Source: three-view drawing plus pictorial views. Frame: mm from the lowest corner of the part. A direction names the side the tool comes from. Give positions to 0.01 mm unless a question says otherwise; leave off trailing zeros. Order: outer loops, then holes, each group sorted by start corner. A loop starts at its lowest first (then second) coordinate and runs counter-clockwise, first axis right, second up. Notation, with made-up numbers: (56, 66) -> (95, 66) arc R21 ccw to (95, 73) -> close; hole circle Ø7 at (74.5, -12). An arc over 180 degrees is marked (long way). Write item = value, one per line.
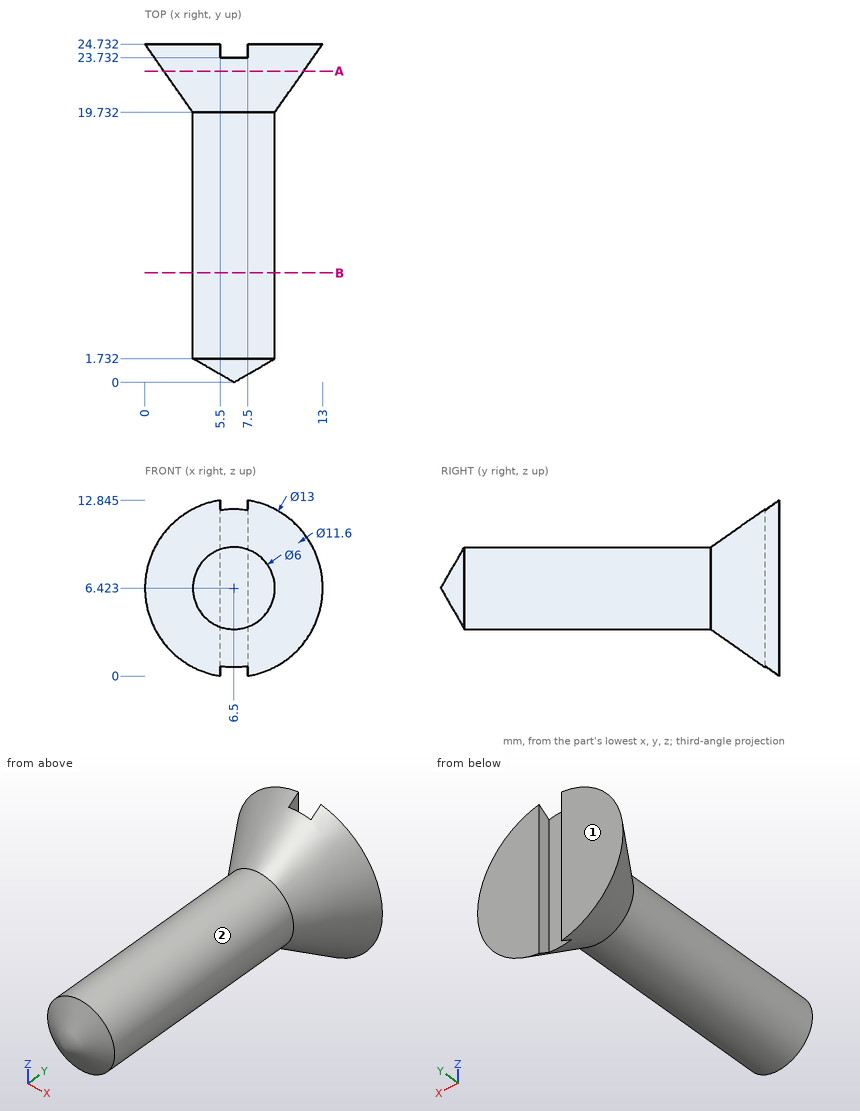
1) First-contact query: P1, Ø0.5, axis at y = 24.5, z = 4, coming from the -X side; P2, Ø5, axis at y = 13.5, z = 6, coming from the -X side; P3, Ø1.1, axis at y = 24, z = 5.5, coming from the +X side; P4, Ø5, axis at x = 11, z = 11.5, coming from the +Y side. Flat tips, straight axial feed; report the tip coordinate or a pass-through.
Check sheet entries:
P1 = 0.43
P2 = 3.5
P3 = 12.81
P4 = 24.73
2) Section query A-A (y = 22.75). Output: boundary loops of the cut face in (x, z) (1 decimal).
Check sheet entries:
outline = circle Ø10.2 at (6.5, 6.4)
3) Section query B-B (y = 8). Output: boundary loops of the cut face in (x, z).
Check sheet entries:
outline = circle Ø6 at (6.5, 6.42)
4) Reachability of the marked faces 1 and 2 from +Z, -Z, +X, -X, +Y, -Y: full face, straight path, thin tool, end or side. Return the list, or none.
Check sheet entries:
face_1 = +Z, -Z, +X, -X, +Y
face_2 = -Y
5) Line query: line 1 (X direction, y = 15.25, z = 6.25) (1 decimal); line 2 (X direction, y = 8.5, z = 7.5); line 3 (Y direction, x = 6, z = 3) (1 decimal). Output: solid intervals per line, ascending. Write a range as from..to.
Check sheet entries:
line_1 = 3.5..9.5
line_2 = 3.7..9.3
line_3 = 20.4..23.7
